from build123d import *

# Parameters (mm, degrees)
SKETCH1_W           = 11
SKETCH1_H           = 11
BOSS_EXTRUDE1_DEPTH = 70
SKETCH2_W           = 11
SKETCH2_H           = 42
BOSS_EXTRUDE2_DEPTH = 12
SKETCH3_W           = 5
SKETCH3_H           = 20
CUT_EXTRUDE1_DEPTH  = 10
CUT_EXTRUDE2_REACH  = 63.53
SKETCH4_R           = 1.7
SKETCH5_W           = 5
SKETCH5_H           = 2
CUT_EXTRUDE3_DEPTH  = 8
SKETCH6_R           = 1.7
CUT_EXTRUDE4_DEPTH  = 17
CUT_EXTRUDE5_START  = -17
SKETCH8_R           = 1.7
CUT_EXTRUDE5_DEPTH  = 17


with BuildPart() as part:
    # Sketch1 → Boss-Extrude1 (new body)
    with BuildSketch(Plane.XY):
        with Locations((5.5, 5.5)):
            Rectangle(SKETCH1_W, SKETCH1_H)
    extrude(amount=BOSS_EXTRUDE1_DEPTH)

    # Sketch2 → Boss-Extrude2 (add)
    with BuildSketch(Plane(origin=(0, 11, 0), x_dir=(1, 0, 0), z_dir=(0, 1, 0))):
        with Locations((5.5, -35)):
            Rectangle(SKETCH2_W, SKETCH2_H)
    extrude(amount=BOSS_EXTRUDE2_DEPTH)

    # Sketch3 → Cut-Extrude1 (cut)
    with BuildSketch(Plane(origin=(0, 23, 0), x_dir=(1, 0, 0), z_dir=(0, 1, 0))):
        with Locations((5.5, -35)):
            Rectangle(SKETCH3_W, SKETCH3_H)
    extrude(amount=-CUT_EXTRUDE1_DEPTH, mode=Mode.SUBTRACT)

    # Cut-Extrude2: up to this face of the body (flat: up to its plane)
    cut_extrude2_end = Plane(part.part.faces().sort_by_distance((5.5, 17, 56))[0])
    # Sketch4 → Cut-Extrude2 (cut, up to the picked face)
    with BuildSketch(Plane(origin=(0, 0, 14), x_dir=(-1, 0, 0), z_dir=(0, 0, -1)), mode=Mode.PRIVATE) as cut_extrude2_sk1:
        with Locations((-5.5, 16.5)):
            Circle(SKETCH4_R)
    cut_extrude2_tool1 = split(extrude(cut_extrude2_sk1.sketch, amount=-CUT_EXTRUDE2_REACH, mode=Mode.PRIVATE), bisect_by=cut_extrude2_end, keep=Keep.BOTH, mode=Mode.PRIVATE)
    add(cut_extrude2_tool1.solids().sort_by(Axis((5.5, 16.5, 14), (0, 0, 1)))[0], mode=Mode.SUBTRACT)

    # Sketch5 → Cut-Extrude3 (cut)
    with BuildSketch(Plane.XZ):
        with Locations((5.5, 55)):
            Rectangle(SKETCH5_W, SKETCH5_H)
        with Locations((5.5, 15)):
            Rectangle(SKETCH5_W, SKETCH5_H)
    extrude(amount=-CUT_EXTRUDE3_DEPTH, mode=Mode.SUBTRACT)

    # Sketch6 → Cut-Extrude4 (cut)
    with BuildSketch(Plane(origin=(0, 0, 0), x_dir=(-1, 0, 0), z_dir=(0, 0, -1))):
        with Locations((-5.5, 5.5)):
            Circle(SKETCH6_R)
    extrude(amount=-CUT_EXTRUDE4_DEPTH, mode=Mode.SUBTRACT)

    # Sketch8 → Cut-Extrude5 (cut)
    with BuildSketch(Plane.XY.offset(70).offset(CUT_EXTRUDE5_START)):
        with Locations(Location((5.5, 5.5, 0), (0, 0, 180))):
            Circle(SKETCH8_R)
    extrude(amount=CUT_EXTRUDE5_DEPTH, mode=Mode.SUBTRACT)


solid = part.part
Build history of the part. All positions in model axes, mm. A direction names the side the tool comes from. Coordinates: 2 decimals unless noted, no trailing zeros. Order: outer loops, then holes, each group sorted by start corner. A loop starts at its lowest first (then second) coordinate and runs counter-clockwise, first axis right, second up. Notation, with made-up numbers: (31.5, 39.25) -> (48.5, 39.25) arc R12 cw to (48.5, 50.25) -> close; hole circle Ø7 at (-2, 17.25). An arc over 180 degrees is marked (long way). One line per item, written item: value.
(1) Slice it at A-A, the plane y = 16.5. List the corners of the cut face in (x, z), plus the area to 3 significant figures.
Checked values:
outline: (0, 14) -> (3.8, 14) -> (3.8, 25) -> (3, 25) -> (3, 45) -> (3.8, 45) -> (3.8, 56) -> (0, 56) -> close; (7.2, 14) -> (11, 14) -> (11, 56) -> (7.2, 56) -> (7.2, 45) -> (8, 45) -> (8, 25) -> (7.2, 25) -> close
area: 287 mm2
(2) Drop flat-ended pins along their axis: pin 1 Ø8 at (y, z) = (20, 34) entering from -X; pin 2 Ø1 at (x, y) = (9, 15.5) entering from +Z; pin 3 Ø3.5 at (x, z) = (6, 65) entering from +Y; pin 4 Ø1.5 at (x, y) = (5, 19) entering from -Z. Give the stop position or say it passes through.
Checked values:
pin 1: x = 0
pin 2: z = 56
pin 3: y = 11
pin 4: z = 14
(3) Mould opens along Z. For faces 1 (the flat face through (3, 18, 35)), 2 (the flat face through (5, 0, 35)), 3 (the flat face through (6, 5, 53)) say: pulls with the +Z half, pulls with the -Z half, needs draft (parallel to the pull), parting line crosses it, or undercut.
Checked values:
face 1: undercut
face 2: needs draft
face 3: pulls with the +Z half
(4) Slice it at D-D, the plane x = 5.5. Count the separate pieces of the cut face and the enclosed holes in it, plus the area to 3 significant figures.
Checked values:
separate pieces: 5
enclosed holes: 0
area: 865 mm2
(5) Probe line 1 (Y direction, x = 5.5, z = 16.35); line 2 (Y direction, x = 5.5, z = 62.25). List the from-to ranges inside material, lowest first. Write a range as [from, to].
Checked values:
line 1: [0, 3.8], [7.2, 14.8], [18.2, 23]
line 2: [0, 3.8], [7.2, 11]
(6) Slice it at B-B, the plane y = 2.75. List the corners of the cut face in (x, z), plus the area to 3 significant figures.
Checked values:
outline: (0, 0) -> (11, 0) -> (11, 70) -> (0, 70) -> close; hole (3, 14) -> (8, 14) -> (8, 16) -> (3, 16) -> close; hole (3, 54) -> (8, 54) -> (8, 56) -> (3, 56) -> close
area: 750 mm2
(7) Tool access for faces 4 (the flat face through (6, 6, 17)), 5 (the cylindrical face through (5.87, 7.16, 53.49)), 6 (the flat face through (5, 13, 35)), 7 (the flat face through (7, 18, 56)), 8 (the flat face through (5, 3, 16)): list every direction of +Z, -Z, +X, -X, +Y, -Y with a clear straight run to the whole face (end or side of a thin tool).
Checked values:
face 4: -Z
face 5: +Z
face 6: +Y
face 7: +Z, +X, -X, +Y
face 8: -Y
(8) Slice it at C-C, the plane x = 8.75. List the corners of the cut face in (y, z), plus the area to 3 significant figures.
Checked values:
outline: (0, 0) -> (11, 0) -> (11, 14) -> (23, 14) -> (23, 56) -> (11, 56) -> (11, 70) -> (0, 70) -> close
area: 1,270 mm2
